Geometry check sheet. Reference: the model listing, model coordinates, mm. Face numbers are marked on the shaded views. Coordinates: 2 decimals unless noted, no trailing zeros. Loops run counter-clockwise (first coordinate to the right, second up) from the corner with the lowest first, then second, coordinate; pieces in that order, holes last. Notation, with made-up numbers: (18, 84) - (42, 84) arc R21 ccw to (42, 112) - close; hole circle Ø1 at (4, -2). An arc over 180 degrees is marked (long way). One line per item, written item: value.
from build123d import *

# Parameters (mm, degrees)
F2_W     = 9
F2_H     = 15
F3_DEPTH = 10.001
F5_D     = 4.2


with BuildPart() as f1:
    # F0 (on Front) → F1 (revolve)
    with BuildSketch(Plane.XZ):
        Polygon((-10, 0), (0, 0), (0, 4), (-10, 5), align=None)
    revolve(axis=Axis((-5, 0, 0), (-1, 0, 0)))

    # F2 (on face) → F3 (intersect, through all)
    with BuildSketch(Plane.YZ):
        Rectangle(F2_W, F2_H)
    extrude(amount=-F3_DEPTH, mode=Mode.INTERSECT)

    # F5 (through all)
    with Locations(Plane.YZ):
        with Locations((0, 0)):
            Hole(F5_D / 2)


solid = f1.part
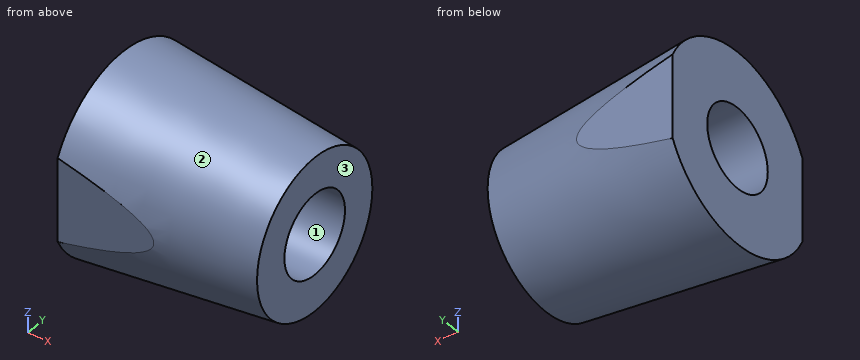
(1) Cross-section at A-A on y = 0. Record the cut outline in (x, z), and give its area (3 significant figures).
Reply:
outline: (-10, -5) - (0, -4) - (0, -2.1) - (-10, -2.1) - close; (-10, 2.1) - (0, 2.1) - (0, 4) - (-10, 5) - close
area: 48.0 mm2
(2) Cross-section at B-B on z = 0. Record the cut outline in (x, y).
Reply:
outline: (-10, -4.5) - (-5, -4.5) - (0, -4) - (0, -2.1) - (-10, -2.1) - close; (-10, 2.1) - (0, 2.1) - (0, 4) - (-5, 4.5) - (-10, 4.5) - close
(3) Material ranges on probe 1 along Z at (x, y) = (-3.25, 0) (3 decimals); probe 2 along Z at (x, y) = (-5, 0); probe 3 along Y at (x, z) = (-6.25, 1.75), recorded low to high. Write a range as from..to.
Reply:
probe 1: -4.325..-2.1, 2.1..4.325
probe 2: -4.5..-2.1, 2.1..4.5
probe 3: -4.28..-1.16, 1.16..4.28
(4) Release check for a two-part mould opening along Z. For the marked faces 1, 2 and 3 record: pulls with the +Z half, pulls with the -Z half, needs draft (parallel to the pull), parting line crosses it, or undercut.
Reply:
face 1: undercut
face 2: parting line crosses it
face 3: needs draft
(5) Cross-section at C-C on x = -8. Record the cut outline in (y, z).
Reply:
outline: (-4.5, -1.67) arc R4.8 ccw to (4.5, -1.67) - (4.5, 1.67) arc R4.8 ccw to (-4.5, 1.67) - close; hole circle Ø4.2 at (0, 0)
(6) Go/stop test with flat-tipped pins: pin 1 Ø1 at (y, z) = (3.5, -1) entering from +X; pin 2 Ø1.5 at (x, z) = (-4, 1) entering from -Y; pin 3 Ø1 at (x, y) = (-5.5, 0.5) entering from +Z; pin 4 Ø4 at (y, z) = (0, 0) entering from -X. Record where each tip stops, or that it passes through.
Reply:
pin 1: x = 0
pin 2: y = -4.43
pin 3: z = 4.59
pin 4: through
(7) Cross-section at D-D on x = -5.75. Record the cut outline in (y, z) (3 decimals).
Reply:
outline: (-4.5, -0.825) arc R4.575 ccw to (4.5, -0.825) - (4.5, 0.825) arc R4.575 ccw to (-4.5, 0.825) - close; hole circle Ø4.2 at (0, 0)
